Input: part model. Units: mm. Frame: model coordinates. A direction names the side the tool comes from. Round coordinates to 2 decimals unless told otherwise and drop trailing zeros. Write each loop counter-clockwise with the first axis right and the second up, starting at its lowest first coordinate (ties: lowest second). Pieces come first, ordered by that corner, then holes. Notation, with made-up numbers: (40.25, 0) - (80.25, 0) arc R33 cw to (80.25, 31) - close; hole circle Ø10 at (-26, 74.5). An arc over 180 degrees is marked (long way). Use one line per item in the form item = value.
```python
from build123d import *

# Parameters (mm, degrees)
SKETCH1_R             = 55
BOSS_EXTRUDE1_DEPTH   = 3
SKETCH9_W             = 40
SKETCH9_H             = 20
BOSS_EXTRUDE4_DEPTH   = 3
SKETCH11_R            = 4.1
CUT_EXTRUDE6_DEPTH    = 4
SKETCH15_R            = 49.7
BOSS_EXTRUDE6_DEPTH   = 3
CHAMFER2_SIZE         = 1
CHAMFER2_SIZE2        = 0.363970234
SKETCH16_W            = 34.7
SKETCH16_H            = 14.7
SKETCH16_R            = 4.1
BOSS_EXTRUDE7_DEPTH   = 9.5
CHAMFER3_SIZE         = 1
CHAMFER3_SIZE2        = 0.363970234
CHAMFER3_PART_2_SIZE  = 1
CHAMFER3_PART_2_SIZE2 = 0.363970234
CHAMFER3_PART_3_SIZE  = 1
CHAMFER3_PART_3_SIZE2 = 0.363970234
CHAMFER3_PART_4_SIZE  = 1
CHAMFER3_PART_4_SIZE2 = 0.363970234


with BuildPart() as part:
    # Sketch1 → Boss-Extrude1 (new body)
    with BuildSketch(Plane(origin=(0, 0, 0), x_dir=(1, 0, 0), z_dir=(0, 1, 0))):
        with Locations(Location((0, 0, 0), (0, 0, 270))):  # turned: the seam where the file's is
            Circle(SKETCH1_R)
    extrude(amount=BOSS_EXTRUDE1_DEPTH)

    # Sketch9 → Boss-Extrude4 (add)
    with BuildSketch(Plane.XZ):
        with Locations((0, 61.23475383)):
            Rectangle(SKETCH9_W, SKETCH9_H)
    extrude(amount=-BOSS_EXTRUDE4_DEPTH)

    # Sketch11 → Cut-Extrude6 (cut, through all)
    with BuildSketch(Plane(origin=(0, 3, 0), x_dir=(1, 0, 0), z_dir=(0, 1, 0))):
        with Locations(Location((-10, -61.23475383, 0), (0, 0, 270))):  # turned: the seam where the file's is
            Circle(SKETCH11_R)
        with Locations(Location((10, -61.23475383, 0), (0, 0, 270))):  # turned: the seam where the file's is
            Circle(SKETCH11_R)
    extrude(amount=-CUT_EXTRUDE6_DEPTH, mode=Mode.SUBTRACT)

    # Sketch15 → Boss-Extrude6 (add)
    with BuildSketch(Plane(origin=(0, 3, 0), x_dir=(1, 0, 0), z_dir=(0, 1, 0))):
        with Locations(Location((0, 0, 0), (0, 0, 270))):  # turned: the seam where the file's is
            Circle(SKETCH15_R)
    extrude(amount=BOSS_EXTRUDE6_DEPTH)

    # Chamfer2
    chamfer2_edges = [part.edges().sort_by_distance(p)[0] for p in [
        (0, 6, -49.7),
    ]]
    chamfer2_side = [part.faces().sort_by_distance(p)[0] for p in [
        (0, 4.5, -49.7),
    ]]
    chamfer(chamfer2_edges, length=CHAMFER2_SIZE, length2=CHAMFER2_SIZE2, reference=chamfer2_side[0])

    # Sketch16 → Boss-Extrude7 (add)
    with BuildSketch(Plane(origin=(0, 3, 0), x_dir=(1, 0, 0), z_dir=(0, 1, 0))):
        with Locations((0, -61.23475383)):
            Rectangle(SKETCH16_W, SKETCH16_H)
        with Locations(Location((-10, -61.23475383, 0), (0, 0, 270))):  # turned: the seam where the file's is
            Circle(SKETCH16_R, mode=Mode.SUBTRACT)
        with Locations(Location((10, -61.23475383, 0), (0, 0, 270))):  # turned: the seam where the file's is
            Circle(SKETCH16_R, mode=Mode.SUBTRACT)
    extrude(amount=BOSS_EXTRUDE7_DEPTH)

    # Chamfer3
    chamfer3_edges = [part.edges().sort_by_distance(p)[0] for p in [
        (-17.35, 12.5, 61.23475383),
    ]]
    chamfer3_side = [part.faces().sort_by_distance(p)[0] for p in [
        (-17.35, 7.75, 61.23475383),
    ]]
    chamfer(chamfer3_edges, length=CHAMFER3_SIZE, length2=CHAMFER3_SIZE2, reference=chamfer3_side[0])

    # Chamfer3 part 2
    chamfer3_part_2_edges = [part.edges().sort_by_distance(p)[0] for p in [
        (0, 12.5, 68.58475383),
    ]]
    chamfer3_part_2_side = [part.faces().sort_by_distance(p)[0] for p in [
        (0, 7.75, 68.58475383),
    ]]
    chamfer(chamfer3_part_2_edges, length=CHAMFER3_PART_2_SIZE, length2=CHAMFER3_PART_2_SIZE2, reference=chamfer3_part_2_side[0])

    # Chamfer3 part 3
    chamfer3_part_3_edges = [part.edges().sort_by_distance(p)[0] for p in [
        (17.35, 12.5, 61.23475383),
    ]]
    chamfer3_part_3_side = [part.faces().sort_by_distance(p)[0] for p in [
        (17.35, 7.75, 61.23475383),
    ]]
    chamfer(chamfer3_part_3_edges, length=CHAMFER3_PART_3_SIZE, length2=CHAMFER3_PART_3_SIZE2, reference=chamfer3_part_3_side[0])

    # Chamfer3 part 4
    chamfer3_part_4_edges = [part.edges().sort_by_distance(p)[0] for p in [
        (0, 12.5, 53.88475383),
    ]]
    chamfer3_part_4_side = [part.faces().sort_by_distance(p)[0] for p in [
        (0, 7.75, 53.88475383),
    ]]
    chamfer(chamfer3_part_4_edges, length=CHAMFER3_PART_4_SIZE, length2=CHAMFER3_PART_4_SIZE2, reference=chamfer3_part_4_side[0])


solid = part.part
```
(1) Draft query along Z for faces 1 (the face through (0, 7, 53.885)), 2 (the face through (2.13, 1.48, -54.96)), 3 (the face through (-1, 0, 9)). Return one class per face: released by +Z, released by -Z, zero draft, split by the parting line, or undercut.
Derived:
face_1 = undercut
face_2 = split by the parting line
face_3 = zero draft
(2) Material intervals for L1, parallel to Y at x = 25, z = 0; L2, parallel to Z at x = 4, y = 3.5; L3, parallel to Z at x = -13, y = 0.5, sorted ascending.
Derived:
L1 = 0 to 6
L2 = -49.54 to 49.54, 53.88 to 68.58
L3 = -53.44 to 58.44, 64.03 to 71.23
(3) First-contact query: pin 1 Ø3.5 at (y, z) = (2, 62) entering from -X; pin 2 Ø1 at (x, y) = (-28, 4.5) entering from +Z; pin 3 Ø4.5 at (y, z) = (6.5, 58.5) entering from +X. Flat tips, straight axial feed; report the tip coordinate or a pass-through.
Derived:
pin_1 = -20
pin_2 = 41.4
pin_3 = 17.35
(4) Cut plane C-C on x = 0. Output: boundary loops of the cut face in (y, z).
Derived:
outline = (0, -55) - (3, -55) - (3, -49.7) - (5, -49.7) - (6, -49.34) - (6, 49.34) - (5, 49.7) - (3, 49.7) - (3, 53.88) - (11.5, 53.88) - (12.5, 54.25) - (12.5, 68.22) - (11.5, 68.58) - (3, 68.58) - (3, 71.23) - (0, 71.23) - close
(5) Cut plane D-D on y = 1.5. Output: boundary loops of the cut face in (x, z).
Derived:
outline = (-20, 51.23) arc R55 ccw (long way) to (20, 51.23) - (20, 71.23) - (-20, 71.23) - close; hole circle Ø8.2 at (-10, 61.23); hole circle Ø8.2 at (10, 61.23)
(6) Access query for faces 4 (the face through (20, 1, 61)), 5 (the face through (-4, 3, 50)), 6 (the face through (0, 7, 68.585)). Directions: +Z, -Z, +X, -X, +Y, -Y. A direction counts if a zero-diameter tool reaches every point of the face in a straight line with its end or side. Return the directions, or none.
Derived:
face_4 = +Z, +X, +Y, -Y
face_5 = +Y
face_6 = +Z, +X, -X, +Y
(7) Cut plane B-B on y = 9.5. Output: boundary loops of the cut face in (x, z).
Derived:
outline = (-17.35, 53.88) - (17.35, 53.88) - (17.35, 68.58) - (-17.35, 68.58) - close; hole circle Ø8.2 at (-10, 61.23); hole circle Ø8.2 at (10, 61.23)
(8) Cut plane A-A on z = 0. Output: boundary loops of the cut face in (x, y).
Derived:
outline = (-55, 0) - (55, 0) - (55, 3) - (49.7, 3) - (49.7, 5) - (49.34, 6) - (-49.34, 6) - (-49.7, 5) - (-49.7, 3) - (-55, 3) - close
